Source: CAD feature listing. Evaluate the final solid. Frame: model axes, mm. Coordinates: 2 decimals unless noted, no trailing zeros. Order: outer loops, then holes, each group sorted by start corner. A loop starts at its lowest first (then second) coordinate and runs counter-clockwise, first axis right, second up.
Item 1: Section A-A on x = 0. Return the cut outline in (y, z) (1 decimal), then the cut area to 3 significant figures.
Item 2: Section C-C on z = 24. Return the cut outline in (x, y).
Item 3: Contact query for flat-ended pins moving along their axis: P1, Ø1, axis at y = -1.5, z = 58.5, coming from the +X side; P2, Ø1, axis at x = 0, z = 43.5, coming from the +Y side; P3, Ø2, axis at y = -1.5, z = 35.5, coming from the -X side. Output: stop coordinate, or through.
Item 4: Ray query, line 1 (Z direction, x = 1, y = 2.25) (1 decimal); line 2 (Y direction, x = 0.25, z = 81); line 3 (Y direction, x = 0.25, z = 78). Return the intervals inside material, ascending.
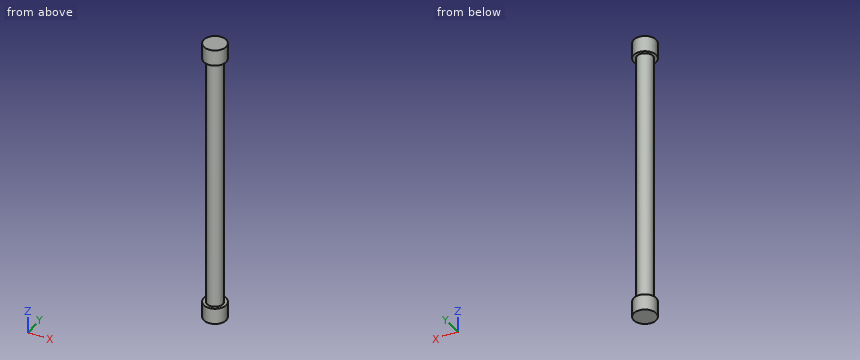
from build123d import *

# Parameters (mm, degrees)
F0_R     = 2.38125
F1_DEPTH = 85.725
F2_R     = 3.33375
F2_R_2   = 2.38125
F3_DEPTH = 4.7625
F4_R     = 3.33375
F4_R_2   = 2.38125
F5_DEPTH = 4.7625


with BuildPart() as f1:
    # F0 (on Top) → F1 (new body)
    with BuildSketch(Plane.XY):
        Circle(F0_R)
    extrude(amount=F1_DEPTH)

    # F2 (on face) → F3 (join)
    with BuildSketch(Plane(origin=(0, 0, 0), x_dir=(1, 0, 0), z_dir=(0, 0, -1))):
        Circle(F2_R)
        Circle(F2_R_2, mode=Mode.SUBTRACT)
    extrude(amount=-F3_DEPTH)

    # F4 (on face) → F5 (join)
    with BuildSketch(Plane.XY.offset(85.725)):
        Circle(F4_R)
        Circle(F4_R_2, mode=Mode.SUBTRACT)
    extrude(amount=-F5_DEPTH)


solid = f1.part
Answer list:
1. outline: (-3.3, 0) - (3.3, 0) - (3.3, 4.8) - (2.4, 4.8) - (2.4, 81) - (3.3, 81) - (3.3, 85.7) - (-3.3, 85.7) - (-3.3, 81) - (-2.4, 81) - (-2.4, 4.8) - (-3.3, 4.8) - close
1. area: 426 mm2
2. outline: circle Ø4.76 at (0, 0)
3. P1: stops at x = 2.16
3. P2: stops at y = 2.38
3. P3: stops at x = -2.33
4. line 1: z = 0 to 4.8, 81 to 85.7
4. line 2: y = -3.32 to 3.32
4. line 3: y = -2.37 to 2.37
